Could you check a few things on this model? Use its own coordinates, in mm. A direction names the side the tool comes from. Give positions to 0.01 mm unless a question says otherwise; leave off trailing zeros. Write each loop counter-clockwise with the first axis right and the second up, starting at its lowest first coordinate (ties: lowest second). Pieces come first, ordered by that corner, then holes. Notation, with made-up numbers: M 33,-22.5 L 39,-22.5 A33 ccw 39,9.5 Z; hole C 53,57 d6. An arc over 180 degrees is marked long. Use one line per item in the form item = value.
from build123d import *

# Parameters (mm, degrees)
SKETCH1_R           = 19.05
BOSS_EXTRUDE1_DEPTH = 104.775
CUT_EXTRUDE1_DEPTH  = 104.775


with BuildPart() as part:
    # Sketch1 → Boss-Extrude1 (new body)
    with BuildSketch(Plane(origin=(0, 0, 0), x_dir=(1, 0, 0), z_dir=(0, 1, 0))):
        Circle(SKETCH1_R)
    extrude(amount=BOSS_EXTRUDE1_DEPTH)

    # Sketch2 → Cut-Extrude1 (cut)
    with BuildSketch(Plane.XZ):
        Polygon((-15.323636661, -1.510781079), (-6.353443536, -14.026049167), (8.970193125, -12.515268087), (15.323636661, 1.510781079), (6.353443536, 14.026049167), (-8.970193125, 12.515268087), align=None)
    extrude(amount=-CUT_EXTRUDE1_DEPTH, mode=Mode.SUBTRACT)

    # Sketch4 → Revolve3 (revolve)
    with BuildSketch(Plane.XY):
        with BuildLine():
            Line((-19.05, 52.3875), (-19.05, 104.775))
            Line((-19.05, 104.775), (-31.75, 104.775))
            ThreePointArc((-31.75, 104.775), (-22.270325917, 79.339958869), (-19.05, 52.3875))
        make_face()
        with BuildLine():
            Line((-19.05, 0), (-19.05, 52.3875))
            ThreePointArc((-19.05, 52.3875), (-22.270325917, 25.435041131), (-31.75, 0))
            Line((-31.75, 0), (-19.05, 0))
        make_face()
    revolve(axis=Axis((0, 0, 0), (0, 1, 0)))


solid = part.part
1) I want a section at A-A, the plane y = 13.5. Please give me the cut outline in (x, z).
Checked values:
outline = C 0,0 d51.72; hole M -15.32,-1.51 L -6.35,-14.03 L 8.97,-12.52 L 15.32,1.51 L 6.35,14.03 L -8.97,12.52 Z
2) For pin 1 Ø10 at (x, y) = (-8.5, 92.5) entering from +Z; pin 2 Ø8 at (x, y) = (20.5, 80.5) entering from -Z; pin 3 Ø1 at (y, z) = (29.5, 18.5) entering from -X, each with a flat end and sliding along its axis, tell me the tip position at first contact or that it passes through.
Checked values:
pin_1 = 27.39
pin_2 = -15.65
pin_3 = -11.53
3) I want a section at B-B, the plane y = 26.5. Please give me the cut outline in (x, z).
Checked values:
outline = C 0,0 d44.04; hole M -15.32,-1.51 L -6.35,-14.03 L 8.97,-12.52 L 15.32,1.51 L 6.35,14.03 L -8.97,12.52 Z
4) For faces 1 (the flat face through (1.2, 51.65, -13.28)), 2 (the flat face through (0, 0, 14)), which set-ups out of +Z, -Z, +X, -X, +Y, -Y let a thin tool reach every point of the face, with its end or its side?
Checked values:
face_1 = +Y, -Y
face_2 = +Z, -Z, +X, -X, -Y
5) Thinking about a two-plate mould opening in X: for faces 3 (the flat face through (-1.2, 51.65, 13.28)), 4 (the flat face through (10.9, 51.65, 7.68)), 5 (the flat face through (0, 104.775, -14)), which applies, released by +X, released by -X, zero draft, split by the parting line, or undercut?
Checked values:
face_3 = undercut
face_4 = undercut
face_5 = zero draft
6) If I drill on L1, parallel to X at y = 21, z = -7; L2, parallel to X at y = 74, z = -8.5; L3, parallel to Z at x = 5, y = 97, over which ranges is the centre line in solid material (lowest first)?
Checked values:
L1 = -22.37 to -11.39, 11.47 to 22.37
L2 = -19.32 to -10.31, 10.79 to 19.32
L3 = -27.66 to -12.91, 13.89 to 27.66
